Source: CAD feature listing. Evaluate the final solid. Frame: model axes, mm. Face numbers are marked on the shaded views. A direction names the side the tool comes from. Give positions to 0.01 mm unless a question says otherwise; leave off trailing zeros. Order: outer loops, then holes, each group sorted by start corner. A loop starts at its lowest first (then second) coordinate and runs counter-clockwise, first axis right, second up. Notation, with made-up numbers: M 36,79 L 90,79 A4 cw 90,84 Z; hole C 14,45.25 d7. An arc over 180 degrees is marked long. Return JSON: item names as keys, results as strings.
Autodesk Inventor part; units mm, degrees
ref_plane "YZ Plane" through (0, 0, 0) normal (1, 0, 0) x (0, 1, 0)
ref_plane "XZ Plane" through (0, 0, 0) normal (0, 1, 0) x (-1, 0, 0)
ref_plane "XY Plane" through (0, 0, 0) normal (0, 0, 1) x (1, 0, 0)
sketch "Эскиз1" plane through (0, 0, 0) normal (1, 0, 0) x (0, 1, 0)
  line L0 (-15, 100) -> (15, 100)
  line L1 (15, 100) -> (15, -100)
  line L2 (15, -100) -> (-15, -100)
  line L3 (-15, -100) -> (-15, 100)
  line L4 (-21, 0) -> (21, 0) construction
  line L5 (0, -140) -> (0, 140) construction
  point P0 (0, 0)
  dimension "d0" = 200
  dimension "d1" = 30
extrude "Выдавливание2" add sketch "Эскиз1" along normal mid plane 59
fillet "Сопряжение1" radius 15 4 edges at (0, 15, 100) (0, -15, 100) (0, 15, -100) (0, -15, -100)
sketch "Эскиз2" plane through (29.5, 0, 0) normal (1, 0, 0) x (0, 0, -1)
  arc A0 (85, -15) -> (85, 15) centre (85, 0) ccw construction
  line L0 (85, 15) -> (-85, 15) construction
  arc A1 (-85, 15) -> (-85, -15) centre (-85, 0) ccw construction
  line L1 (-85, -15) -> (85, -15) construction
  line L2 (-99, -14) -> (99, -14)
  line L3 (99, -14) -> (99, 14)
  line L4 (99, 14) -> (-99, 14)
  line L5 (-99, 14) -> (-99, -14)
  arc A2 (-85, 14) -> (-99, 0) centre (-85, 0) ccw
  arc A3 (-85, 15) -> (-85, -15) centre (-85, 0) ccw
  arc A4 (-99, 0) -> (-85, -14) centre (-85, 0) ccw
  arc A5 (99, 0) -> (85, 14) centre (85, 0) ccw
  arc A6 (85, -15) -> (85, 15) centre (85, 0) ccw
  arc A7 (85, -14) -> (99, 0) centre (85, 0) ccw
  point P0 (0, 0)
  dimension "d11" = 198
  dimension "d12" = 28
  dimension "d13" = 1
  dimension "d14" = 1
extrude "Выдавливание3" cut sketch "Эскиз2" against normal blind 59 contours A4 A2 L4 A5 A7 L2
properties part number "Лента конвейера"
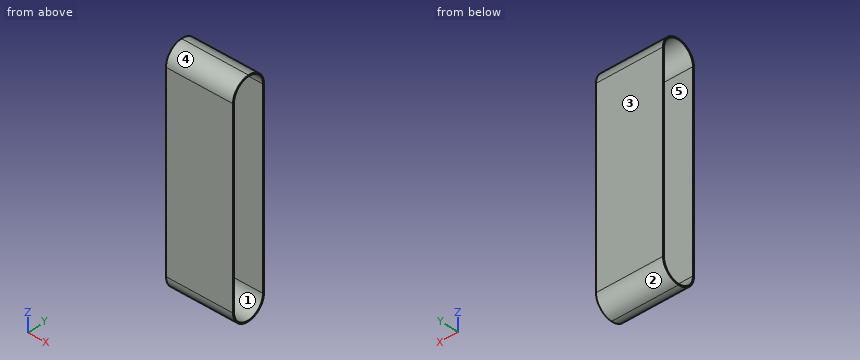
1. Set-up query: the marked faces 4 and 5. Return all of +Z, -Z, +X, -X, +Y, -Y with unobstructed straight access to the full face (end or side cutting, diameter ignored); none if empty.
Evaluation:
{"face 4": "+Z, +X, -X, -Y", "face 5": "+X, -X"}
2. Draft query along Z for the marked faces 1, 2 and 3. Return one class per face: pulls with the +Z half, pulls with the -Z half, needs draft (parallel to the pull), parting line crosses it, or undercut.
Evaluation:
{"face 1": "undercut", "face 2": "pulls with the -Z half", "face 3": "needs draft"}
3. Ray query, probe 1 along Y at (x, z) = (17.5, -44); probe 2 along Z at (x, y) = (-6, -0.25); probe 3 along Z at (x, y) = (-22.5, 8). Return the intervals inside material, ascending.
Evaluation:
{"probe 1": "y = -15 to -14, 14 to 15", "probe 2": "z = -100 to -99, 99 to 100", "probe 3": "z = -97.69 to -96.49, 96.49 to 97.69"}
4. First-contact query: pin 1 (1.5 mm diameter, centred on x = 5, y = -6, fed in from -Z); pin 2 (5 mm diameter, centred on x = -1, y = 10.5, fed in from +Z). Flat tips, straight axial feed; report the tip coordinate or a pass-through.
Evaluation:
{"pin 1": "stops at z = -99.05", "pin 2": "stops at z = 97.69"}
5. Section query B-B (y = 2). Return loops of the section in (x, z).
Evaluation:
{"outline": "M -29.5,-99.87 L 29.5,-99.87 L 29.5,-98.86 L -29.5,-98.86 Z; M -29.5,98.86 L 29.5,98.86 L 29.5,99.87 L -29.5,99.87 Z"}
6. Section query A-A (z = -79). Return loops of the section in (x, y).
Evaluation:
{"outline": "M -29.5,-15 L 29.5,-15 L 29.5,-14 L -29.5,-14 Z; M -29.5,14 L 29.5,14 L 29.5,15 L -29.5,15 Z"}
